Answer from the drawing. Dimensions are ordinates in mm from the lowest x, y and z of the part. A direction names the side the tool comes from. Round coordinates to 2 decimals unless told otherwise and drop trailing zeros. Order: outer loops, then holes, each group sorted by start corner. A loop starts at its lowest first (then second) coordinate and runs counter-clockwise, first axis right, second up. Notation, with made-up numbers: M -33.5,-15 L -0.5,-15 A12 ccw -0.5,7 Z; hole C -15.5,69.25 d4. An arc over 180 degrees is marked long. Write item = value, one per line. Start each with the question number.
(1) For a pull along X with two mould halves and no side action, classify the marked faces 5, 6 and 7 as released by +X, released by -X, zero draft, split by the parting line, or undercut.
(2) Straight lines are drawn through the part: probe 1 along X at (y, z) = (32, 13); probe 2 along X at (y, z) = (38.5, 60.5); probe 3 along Y at (x, z) = (146, 11). For each, find the intervals that lie inside material, in ascending order. Write a range as from..to.
(3) A cutting plane is placed at B-B, the plane y = 55. Determine the outline of the cut face in (x, z), and give its area (3 significant figures).
(4) Each of these flat-tipped pins is pushed along its axis until it touches: pin 1 (2 mm diameter, centred on y = 36.5, z = 13, fed in from +X); pin 2 (3 mm diameter, centred on x = 82, z = 25.5, fed in from -Y) (1 decimal); pin 3 (22.5 mm diameter, centred on y = 32.5, z = 46, fed in from +X). Where does it stop, or does it pass through?
(5) A cutting plane is placed at D-D, the plane y = 12. Determine the outline of the cut face in (x, z), and give its area (3 significant figures).
(6) Which of the six approach directions +Z, -Z, +X, -X, +Y, -Y give full straight-line access (tool end or side, diameter ignored) to the marked faces 1, 2, 3 and 4?
(7) A cutting plane is placed at C-C, the plane z = 26. Determine the outline of the cut face in (x, y).
(8) A cutting plane is placed at A-A, the plane x = 81. Determine the outline of the cut face in (y, z), and give its area (3 significant figures).
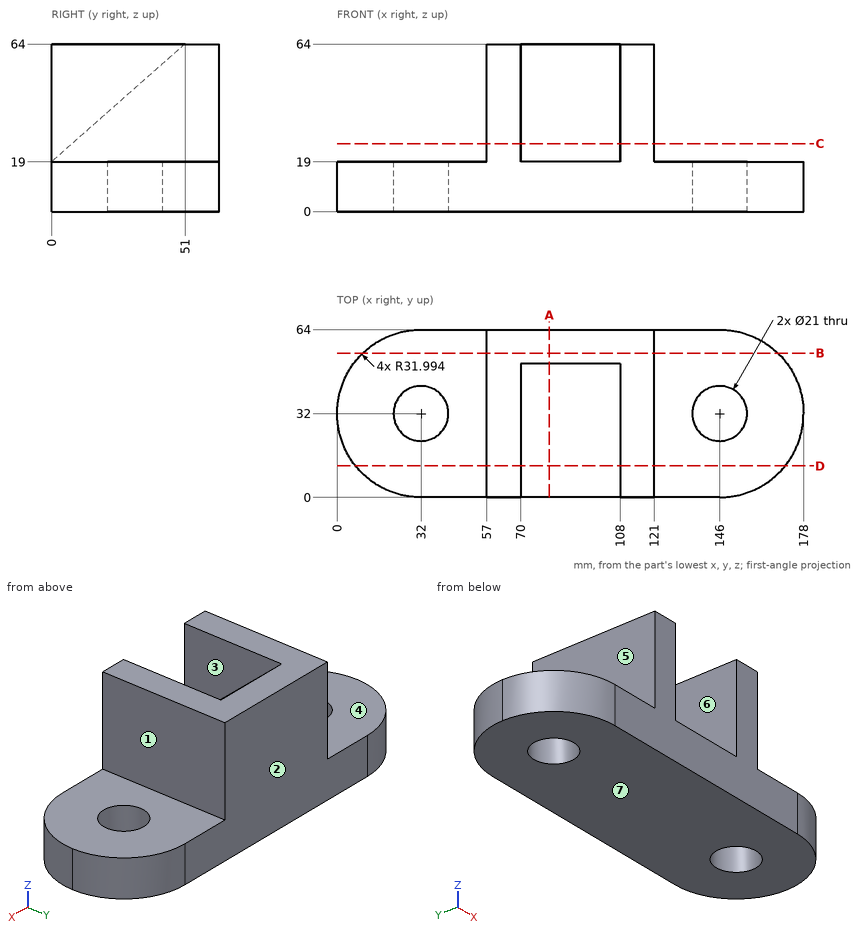
Reported:
q1.face_5 = released by -X
q1.face_6 = undercut
q1.face_7 = zero draft
q2.probe_1 = 0..21.5, 42.5..135.5, 156.5..178
q2.probe_2 = 57..70, 108..121
q2.probe_3 = 0..21.5, 42.5..64
q3.outline = M 9.75,0 L 168.25,0 L 168.25,19 L 121,19 L 121,64 L 57,64 L 57,19 L 9.75,19 Z
q3.area = 5,890 mm²
q4.pin_1 = 177.81
q4.pin_2 = 5.7
q4.pin_3 = 121
q5.outline = M 7.02,0 L 170.98,0 L 170.98,19 L 121,19 L 121,64 L 108,64 L 108,29.59 L 70,29.59 L 70,64 L 57,64 L 57,19 L 7.02,19 Z
q5.area = 4,690 mm²
q6.face_1 = +Z, +X, +Y, -Y
q6.face_2 = +Z, -Z, +X, -X, +Y
q6.face_3 = +Z, -Y
q6.face_4 = +Z, -X, +Y, -Y
q7.outline = M 57,0 L 70,0 L 70,7.93 L 108,7.93 L 108,0 L 121,0 L 121,64 L 57,64 Z
q8.outline = M 0,0 L 64,0 L 64,64 L 51,64 L 0,19 Z
q8.area = 2,950 mm²
